Can you work these out from the model? Positions are in its coordinate system, mm. A direction names the side the tool comes from. Coordinates: 2 decimals unless noted, no trailing zeros. Write each loop counter-clockwise with the first axis right and the second up, starting at its lowest first coordinate (ties: lowest second). Pieces come first, ordered by that corner, then holes. Notation, with made-up numbers: M -12,50 L 36,50 A15 ccw 36,75 Z; hole C -17.75,-27 d6. An arc over 180 degrees is marked long. Use one line per item in the form item = value. Start each with the question number.
```python
from build123d import *

# Parameters (mm, degrees)
SKETCH1_W           = 20
SKETCH1_H           = 10
SKETCH1_R           = 1.65
BOSS_EXTRUDE1_DEPTH = 5
SKETCH2_W           = 20
SKETCH2_H           = 7
BOSS_EXTRUDE2_DEPTH = 18
BOSS_EXTRUDE3_DEPTH = 3.175
BOSS_EXTRUDE4_START = 12
SKETCH4_R           = 4
BOSS_EXTRUDE4_DEPTH = 12


with BuildPart() as part:
    # Sketch1 → Boss-Extrude1 (new body)
    with BuildSketch(Plane(origin=(0, 0, 0), x_dir=(0, 0, -1), z_dir=(1, 0, 0))):
        Rectangle(SKETCH1_W, SKETCH1_H)
        with Locations((-5, 0)):
            Circle(SKETCH1_R, mode=Mode.SUBTRACT)
        with Locations((5, 0)):
            Circle(SKETCH1_R, mode=Mode.SUBTRACT)
    extrude(amount=BOSS_EXTRUDE1_DEPTH)

    # Sketch2 → Boss-Extrude2 (add)
    with BuildSketch(Plane(origin=(5, 0, 0), x_dir=(0, 0, -1), z_dir=(1, 0, 0))):
        with Locations((0, 1.5)):
            Rectangle(SKETCH2_W, SKETCH2_H)
    extrude(amount=BOSS_EXTRUDE2_DEPTH)

    # Sketch3 → Boss-Extrude3 (add)
    with BuildSketch(Plane(origin=(23, 0, 0), x_dir=(0, 0, -1), z_dir=(1, 0, 0))):
        with BuildLine():
            Line((10, 5), (-10, 5))
            Line((-10, 5), (-10, -2))
            Line((-10, -2), (-0.770329614, -2))
            Line((-0.770329614, -2), (6, -2))
            ThreePointArc((6, -2), (7.171572875, 0.828427125), (10, 2))
            Line((10, 2), (10, 2.308131846))
            Line((10, 2.308131846), (10, 5))
        make_face()
        with BuildLine():
            Line((10, -2), (10, 2))
            ThreePointArc((10, 2), (7.171572875, 0.828427125), (6, -2))
            Line((6, -2), (10, -2))
        make_face()
        with BuildLine():
            ThreePointArc((11.485562705, 1.713906764), (10.756430085, 1.927825547), (10, 2))
            Line((10, 2), (10, -2))
            Line((10, -2), (6, -2))
            ThreePointArc((6, -2), (6.687731078, -4.242515237), (8.514437295, -5.713906764))
            Line((8.514437295, -5.713906764), (28.514437295, -13.713906764))
            ThreePointArc((28.514437295, -13.713906764), (33.713906764, -11.485562705), (31.485562705, -6.286093236))
            Line((31.485562705, -6.286093236), (11.485562705, 1.713906764))
        make_face()
        with BuildLine():
            Line((6, -2), (-0.770329614, -2))
            Line((-0.770329614, -2), (8.514437295, -5.713906764))
            ThreePointArc((8.514437295, -5.713906764), (6.687731078, -4.242515237), (6, -2))
        make_face()
        with BuildLine():
            Line((11.485562705, 1.713906764), (10, 2.308131846))
            Line((10, 2.308131846), (10, 2))
            ThreePointArc((10, 2), (10.756430085, 1.927825547), (11.485562705, 1.713906764))
        make_face()
    extrude(amount=BOSS_EXTRUDE3_DEPTH)

    # Sketch4 → Boss-Extrude4 (add)
    with BuildSketch(Plane.ZY.offset(-23).offset(BOSS_EXTRUDE4_START)):
        with Locations((-30, -10)):
            Circle(SKETCH4_R)
    extrude(amount=-BOSS_EXTRUDE4_DEPTH)


solid = part.part
```
1) Suppose I cut it at B-B on y = -3. Please give me the cut outline in (x, z) (3 decimals), and give its area (3 significant figures).
2) Suppose I cut it at D-D on y = 0. Please give me the cut outline in (x, z) (3 decimals), and give its area (3 significant figures).
3) Which directions (+Z, -Z, +X, -X, +Y, -Y) give clear straight access to the entire face, cutting with the end or side of a thin tool? Please do faces 1 (the face through (0, 0, 0)), 2 (the face through (5, -3, 0)), 3 (the face through (5, 0, 5)).
4) Please list where these lines run through material, in increasing order: line 1 (Y direction, x = 1.65, z = 5); line 2 (Y direction, x = 2.25, z = -7.5); line 3 (Y direction, x = 19, z = -8).
5) If we mould it in two halves opening along Z, with no side actions, what happens to faces 4 (the face through (2.46, 0.07, -3.35)), 5 (the face through (13, 5, 0)), 6 (the face through (10, 1, -10)), 7 (the face through (13, 1, 10))? For each: +Z half, -Z half, draft (parallel to the pull), parting line (faces both ways), or undercut.
6) Suppose I cut it at C-C on z = -5. Please give me the cut outline in (x, y) (3 decimals).
7) Suppose I cut it at A-A on x = 12.5. Please give me the cut outline in (y, z).
8) Will these pins go through, and if not, where does the flat tip stop? pin 1 Ø5 at (y, z) = (-0.5, -24) entering from -X; pin 2 Ø1.6 at (y, z) = (0.5, -5) entering from -X; pin 3 Ø6 at (x, z) = (10.5, -8.5) entering from -Y; pin 4 Ø1.5 at (x, z) = (2, 2) entering from -Y.
Computed values:
q1.outline = M 0,-10 L 5,-10 L 5,10 L 0,10 Z; M 23,-23.27 L 26.175,-23.27 L 26.175,-1.73 L 23,-1.73 Z
q1.area = 168 mm²
q2.outline = M 0,-10 L 23,-10 L 23,-15.77 L 26.175,-15.77 L 26.175,10 L 0,10 L 0,6.65 L 5,6.65 L 5,3.35 L 0,3.35 L 0,-3.35 L 5,-3.35 L 5,-6.65 L 0,-6.65 Z
q2.area = 509 mm²
q3.face_1 = +Z, -Z, -X, +Y, -Y
q3.face_2 = +Z, -Z, -Y
q3.face_3 = -X
q4.line_1 = -5 to -1.65, 1.65 to 5
q4.line_2 = -5 to 5
q4.line_3 = -2 to 5
q5.face_4 = undercut
q5.face_5 = draft
q5.face_6 = -Z half
q5.face_7 = +Z half
q6.outline = M 0,-5 L 5,-5 L 5,-2 L 23,-2 L 23,-4.308 L 26.175,-4.308 L 26.175,5 L 0,5 L 0,1.65 L 5,1.65 L 5,-1.65 L 0,-1.65 Z
q7.outline = C -10,-30 d8; M -2,-10 L 5,-10 L 5,10 L -2,10 Z
q8.pin_1 = through
q8.pin_2 = 5
q8.pin_3 = -2
q8.pin_4 = -5
